Input: part model. Units: mm. Frame: model coordinates. A direction names the side the tool comes from. Round coordinates to 2 decimals unless told otherwise and drop trailing zeros. Write each loop counter-clockwise with the first axis right and the second up, starting at its lowest first coordinate (ties: lowest second). Pieces come first, ordered by that corner, then holes. Notation, with made-up numbers: (60, -18) - (105, -18) arc R20 ccw to (105, -10) - close; hole circle Ø7 at (34.5, 14.5). An arc over 180 degrees is marked (long way). Use one line per item in the form item = value.
```python
from build123d import *

# Parameters (mm, degrees)
SKETCH1_W           = 30.48
SKETCH1_H           = 33.782
BOSS_EXTRUDE1_DEPTH = 5.08
SKETCH2_R           = 2.54
BOSS_EXTRUDE2_DEPTH = 1.5875
SKETCH3_W           = 5.842
SKETCH3_H           = 10.16
BOSS_EXTRUDE3_DEPTH = 0.9525
SKETCH4_W           = 10.16
SKETCH4_H           = 5.842
BOSS_EXTRUDE4_DEPTH = 0.9525
SKETCH5_W           = 6.35
SKETCH5_H           = 2.131234452
BOSS_EXTRUDE5_DEPTH = 7.62


with BuildPart() as part:
    # Sketch1 → Boss-Extrude1 (new body, symmetric)
    with BuildSketch(Plane(origin=(0, 0, 0), x_dir=(1, 0, 0), z_dir=(0, 1, 0))):
        Rectangle(SKETCH1_W, SKETCH1_H)
    extrude(amount=BOSS_EXTRUDE1_DEPTH, both=True)

    # Sketch2 → Boss-Extrude2 (add, symmetric)
    with BuildSketch(Plane.XY.offset(16.891)):
        with Locations((-8.636, 0)):
            Circle(SKETCH2_R)
    extrude(amount=BOSS_EXTRUDE2_DEPTH, both=True)

    # Sketch3 → Boss-Extrude3 (add, symmetric)
    with BuildSketch(Plane(origin=(0, 0, 0), x_dir=(1, 0, 0), z_dir=(0, 1, 0))):
        with Locations((18.161, -11.811)):
            Rectangle(SKETCH3_W, SKETCH3_H)
        with BuildLine():
            Line((19.304, -8.636), (19.304, -14.986))
            ThreePointArc((19.304, -14.986), (18.161, -16.129), (17.018, -14.986))
            Line((17.018, -14.986), (17.018, -8.636))
            ThreePointArc((17.018, -8.636), (18.161, -7.493), (19.304, -8.636))
        make_face(mode=Mode.SUBTRACT)
    boss_extrude3 = extrude(amount=BOSS_EXTRUDE3_DEPTH, both=True)

    # Mirror1: Boss-Extrude3 across plane
    add(boss_extrude3.mirror(Plane(origin=(0, 0, 0), x_dir=(0, 0, 1), z_dir=(1, 0, 0))))

    # Sketch4 → Boss-Extrude4 (add, symmetric)
    with BuildSketch(Plane(origin=(0, 0, 0), x_dir=(1, 0, 0), z_dir=(0, 1, 0))):
        with Locations((0, 19.812)):
            Rectangle(SKETCH4_W, SKETCH4_H)
        with BuildLine():
            Line((-3.175, 20.955), (3.175, 20.955))
            ThreePointArc((3.175, 20.955), (4.318, 19.812), (3.175, 18.669))
            Line((3.175, 18.669), (-3.175, 18.669))
            ThreePointArc((-3.175, 18.669), (-4.318, 19.812), (-3.175, 20.955))
        make_face(mode=Mode.SUBTRACT)
    extrude(amount=BOSS_EXTRUDE4_DEPTH, both=True)

    # Sketch5 → Boss-Extrude5 (add)
    with BuildSketch(Plane.ZY.offset(15.24)):
        with Locations((-7.62, 0)):
            Rectangle(SKETCH5_W, SKETCH5_H)
    extrude(amount=BOSS_EXTRUDE5_DEPTH)


solid = part.part
```
(1) Cut plane A-A on y = 0. Count the separate pieces of the cut face and the enclosed holes in it, then the cut area to 3 significant figures.
Derived:
separate_pieces = 1
enclosed_holes = 3
area = 1,210 mm^2
(2) Access query for faces 1 (the face through (-19, -1.066, -8)), 2 (the face through (-16.8, 0.952, 11.7)), 3 (the face through (-17.018, 0, 12)). Directions: +Z, -Z, +X, -X, +Y, -Y. A direction counts if a zero-diameter tool reaches every point of the face in a straight line with its end or side. Return the directions, or none.
Derived:
face_1 = +Z, -Z, -X, -Y
face_2 = +Z, -X, +Y
face_3 = +Y, -Y
(3) First-contact query: pin 1 Ø3 at (x, z) = (-1, -21) entering from +Y; pin 2 Ø1.8 at (x, z) = (-19, 14) entering from -Y; pin 3 Ø3 at (x, z) = (-17.5, -6.5) entering from +Y. Flat tips, straight axial feed; report the tip coordinate or a pass-through.
Derived:
pin_1 = 0.95
pin_2 = -0.95
pin_3 = 1.07
(4) Cut plane C-C on x = 12. Output: boundary loops of the cut face in (y, z), then the cut area to 3 significant figures.
Derived:
outline = (-5.08, -16.89) - (5.08, -16.89) - (5.08, 16.89) - (-5.08, 16.89) - close
area = 343 mm^2
(5) Cut plane B-B on z = -3.5. Output: boundary loops of the cut face in (x, y).
Derived:
outline = (-15.24, -5.08) - (15.24, -5.08) - (15.24, 5.08) - (-15.24, 5.08) - close
(6) Draft query along X for faces 4 (the face through (0, 5.08, 0)), 5 (the face through (-19.304, 0, 12)), 6 (the face through (-21.082, 0, 12)). Return one class per face: released by +X, released by -X, zero draft, split by the parting line, or undercut.
Derived:
face_4 = zero draft
face_5 = undercut
face_6 = released by -X
(7) Material intervals for L1, parallel to Z at x = -1.5, y = 1.5; L2, parallel to X at y = 2.75, z = 13; L3, parallel to X at y = -0.5, z = -20.5, sorted ascending.
Derived:
L1 = -16.89 to 16.89
L2 = -15.24 to 15.24
L3 = -5.08 to -4.09, 4.09 to 5.08
